Verification items for the finished model (mm, model axes). Face numbers are marked on the shaded views. Round coordinates to 2 decimals unless told otherwise and drop trailing zeros. Order: outer loops, then holes, each group sorted by start corner. A loop starts at its lowest first (then second) coordinate and runs counter-clockwise, first axis right, second up. Notation, with made-up numbers: (25.25, -25) -> (54.25, -25) arc R30 ccw to (54.25, -1) -> close; hole circle Ø3 at (81, 35). An arc over 180 degrees is marked (long way). Return JSON: item names as keys, results as strings. Group by question number.
1) Draft check along Y on the marked faces 1, 2, 3 and 4. Enter one of: pulls with the +Y half, pulls with the -Y half, needs draft (parallel to the pull), parting line crosses it, or undercut.
2) Section check A-A on y = 49.5. Enter the section's corners in (x, z) (3 decimals).
3) Scan lines: L1, parallel to Z at x = 2.25, y = 44 (3 decimals); L2, parallel to Z at x = 3.75, y = 17; L3, parallel to Y at x = 4.25, z = 9. Record each from-to range of solid material in increasing order.
4) Depth check by flat-ended pin: pin 1 (0.5 mm diameter, centred on x = 4, z = 3.5, fed in from +Y); pin 2 (4 mm diameter, centred on y = 18.5, z = 18, fed in from +X); pin 3 (1 mm diameter, centred on x = 6, z = 19.5, fed in from -Y); pin 4 (0.5 mm diameter, centred on x = 4, y = 17, fed in from -Z). Enter the tip coordinate at first touch or a pass-through.
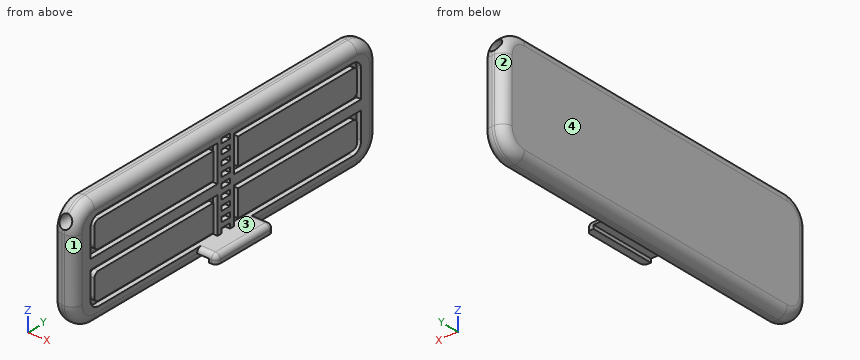
```python
from build123d import *

# Parameters (mm, degrees)
F1_DEPTH     = 4.5
F2_R         = 1.225
F3_DEPTH     = 74
F4_T1_DEPTH  = 64
F4_T3_DEPTH  = 13
F4_T6_ANGLE  = 90
F4_T8_ANGLE  = 90
F4_T10_ANGLE = 90
F4_T12_ANGLE = 90
F4_T14_ANGLE = 90
F4_T16_ANGLE = 90
F4_T18_ANGLE = 90
F4_T20_ANGLE = 90
F6_DEPTH     = 1
F7_W         = 2
F7_H         = 1
F8_DEPTH     = 1
F10_DEPTH    = 1
F11_W        = 14
F11_H        = 1
F12_DEPTH    = 4
F13_W        = 1.5
F13_H        = 14
F14_DEPTH    = 0.75
F15_R        = 0.99999


# Not quite as in the source:
# - a fillet or chamfer that OpenCascade refuses, or shapes differently, is made with other operations: its cross-section is extruded or revolved along the edge and cut away or added
# - a fillet or chamfer is up to 0.001 mm smaller than in the source, because OpenCascade refuses the exact size


with BuildPart() as f1:
    # F0 (on Right) → F1 (new body)
    with BuildSketch(Plane.YZ):
        with BuildLine():
            ThreePointArc((0, 5), (1.4644660941, 1.4644660941), (5, 0))
            Line((5, 0), (69, 0))
            ThreePointArc((69, 0), (72.5355339059, 1.4644660941), (74, 5))
            Line((74, 5), (74, 18))
            ThreePointArc((74, 18), (72.5355339059, 21.5355339059), (69, 23))
            Line((69, 23), (5, 23))
            ThreePointArc((5, 23), (1.4644660941, 21.5355339059), (0, 18))
            Line((0, 18), (0, 5))
        make_face()
    extrude(amount=F1_DEPTH)

    # F2 (on face) → F3 (cut, through all)
    with BuildSketch(Plane(origin=(0, 74, 0), x_dir=(-1, 0, 0), z_dir=(0, 1, 0))):
        with Locations((-2.25, 20)):
            Circle(F2_R)
    extrude(amount=-F3_DEPTH, mode=Mode.SUBTRACT)

    # F4: fillet of radius 2 on 16 edges, made by hand

    # F4_s2 → F4_t1 (cut)
    with BuildSketch(Plane.XZ.offset(-69)):
        with BuildLine():
            ThreePointArc((0, 21), (0.5857864376, 22.4142135624), (2, 23))
            Line((2, 23), (0, 23))
            Line((0, 23), (0, 21))
        make_face()
        with BuildLine():
            ThreePointArc((4.5, 21), (3.9142135624, 22.4142135624), (2.5, 23))
            Line((2.5, 23), (4.5, 23))
            Line((4.5, 23), (4.5, 21))
        make_face()
        with BuildLine():
            ThreePointArc((2, 0), (0.5857864376, 0.5857864376), (0, 2))
            Line((0, 2), (0, 0))
            Line((0, 0), (2, 0))
        make_face()
        with BuildLine():
            ThreePointArc((2.5, 0), (3.9142135624, 0.5857864376), (4.5, 2))
            Line((4.5, 2), (4.5, 0))
            Line((4.5, 0), (2.5, 0))
        make_face()
    extrude(amount=F4_T1_DEPTH, mode=Mode.SUBTRACT)

    # F4_s4 → F4_t3 (cut)
    with BuildSketch(Plane.XY.offset(5)):
        with BuildLine():
            ThreePointArc((2, 0), (0.5857864376, 0.5857864376), (0, 2))
            Line((0, 2), (0, 0))
            Line((0, 0), (2, 0))
        make_face()
        with BuildLine():
            ThreePointArc((2.5, 0), (3.9142135624, 0.5857864376), (4.5, 2))
            Line((4.5, 2), (4.5, 0))
            Line((4.5, 0), (2.5, 0))
        make_face()
        with BuildLine():
            ThreePointArc((0, 72), (0.5857864376, 73.4142135624), (2, 74))
            Line((2, 74), (0, 74))
            Line((0, 74), (0, 72))
        make_face()
        with BuildLine():
            ThreePointArc((4.5, 72), (3.9142135624, 73.4142135624), (2.5, 74))
            Line((2.5, 74), (4.5, 74))
            Line((4.5, 74), (4.5, 72))
        make_face()
    extrude(amount=F4_T3_DEPTH, mode=Mode.SUBTRACT)

    # F4_s5 → F4_t6 (revolve, cut)
    with BuildSketch(Plane.XY.offset(5)):
        with BuildLine():
            ThreePointArc((2, 0), (0.5857864376, 0.5857864376), (0, 2))
            Line((0, 2), (0, 0))
            Line((0, 0), (2, 0))
        make_face()
    revolve(axis=Axis((0, 5, 5), (1, 0, 0)), revolution_arc=F4_T6_ANGLE, mode=Mode.SUBTRACT)

    # F4_s7 → F4_t8 (revolve, cut)
    with BuildSketch(Plane.XY.offset(5)):
        with BuildLine():
            ThreePointArc((2.5, 0), (3.9142135624, 0.5857864376), (4.5, 2))
            Line((4.5, 2), (4.5, 0))
            Line((4.5, 0), (2.5, 0))
        make_face()
    revolve(axis=Axis((4.5, 5, 5), (1, 0, 0)), revolution_arc=F4_T8_ANGLE, mode=Mode.SUBTRACT)

    # F4_s9 → F4_t10 (revolve, cut)
    with BuildSketch(Plane.XZ.offset(-69)):
        with BuildLine():
            ThreePointArc((0, 2), (0.5857864376, 0.5857864376), (2, 0))
            Line((2, 0), (0, 0))
            Line((0, 0), (0, 2))
        make_face()
    revolve(axis=Axis((0, 69, 5), (1, 0, 0)), revolution_arc=F4_T10_ANGLE, mode=Mode.SUBTRACT)

    # F4_s11 → F4_t12 (revolve, cut)
    with BuildSketch(Plane.XY.offset(18)):
        with BuildLine():
            ThreePointArc((0, 72), (0.5857864376, 73.4142135624), (2, 74))
            Line((2, 74), (0, 74))
            Line((0, 74), (0, 72))
        make_face()
    revolve(axis=Axis((0, 69, 18), (1, 0, 0)), revolution_arc=F4_T12_ANGLE, mode=Mode.SUBTRACT)

    # F4_s13 → F4_t14 (revolve, cut)
    with BuildSketch(Plane.XZ.offset(-5)):
        with BuildLine():
            ThreePointArc((0, 21), (0.5857864376, 22.4142135624), (2, 23))
            Line((2, 23), (0, 23))
            Line((0, 23), (0, 21))
        make_face()
    revolve(axis=Axis((0, 5, 18), (1, 0, 0)), revolution_arc=F4_T14_ANGLE, mode=Mode.SUBTRACT)

    # F4_s15 → F4_t16 (revolve, cut)
    with BuildSketch(Plane.XZ.offset(-69)):
        with BuildLine():
            ThreePointArc((4.5, 2), (3.9142135624, 0.5857864376), (2.5, 0))
            Line((2.5, 0), (4.5, 0))
            Line((4.5, 0), (4.5, 2))
        make_face()
    revolve(axis=Axis((4.5, 69, 5), (1, 0, 0)), revolution_arc=F4_T16_ANGLE, mode=Mode.SUBTRACT)

    # F4_s17 → F4_t18 (revolve, cut)
    with BuildSketch(Plane.XY.offset(18)):
        with BuildLine():
            ThreePointArc((4.5, 72), (3.9142135624, 73.4142135624), (2.5, 74))
            Line((2.5, 74), (4.5, 74))
            Line((4.5, 74), (4.5, 72))
        make_face()
    revolve(axis=Axis((4.5, 69, 18), (1, 0, 0)), revolution_arc=F4_T18_ANGLE, mode=Mode.SUBTRACT)

    # F4_s19 → F4_t20 (revolve, cut)
    with BuildSketch(Plane.XZ.offset(-5)):
        with BuildLine():
            ThreePointArc((4.5, 21), (3.9142135624, 22.4142135624), (2.5, 23))
            Line((2.5, 23), (4.5, 23))
            Line((4.5, 23), (4.5, 21))
        make_face()
    revolve(axis=Axis((4.5, 5, 18), (1, 0, 0)), revolution_arc=F4_T20_ANGLE, mode=Mode.SUBTRACT)

    # F5 (on face) → F6 (cut)
    with BuildSketch(Plane.YZ.offset(4.5)):
        with BuildLine():
            Line((35, 20), (6, 20))
            ThreePointArc((6, 20), (4.5857864376, 19.4142135624), (4, 18))
            Line((4, 18), (4, 12.5))
            Line((4, 12.5), (35, 12.5))
            Line((35, 12.5), (35, 20))
        make_face()
        with BuildLine():
            ThreePointArc((4, 5), (4.5857864376, 3.5857864376), (6, 3))
            Line((6, 3), (35, 3))
            Line((35, 3), (35, 10.5))
            Line((35, 10.5), (4, 10.5))
            Line((4, 10.5), (4, 5))
        make_face()
        with BuildLine():
            Line((68, 20), (39, 20))
            Line((39, 20), (39, 12.5))
            Line((39, 12.5), (70, 12.5))
            Line((70, 12.5), (70, 18))
            ThreePointArc((70, 18), (69.4142135624, 19.4142135624), (68, 20))
        make_face()
        with BuildLine():
            Line((39, 10.5), (39, 3))
            Line((39, 3), (68, 3))
            ThreePointArc((68, 3), (69.4142135624, 3.5857864376), (70, 5))
            Line((70, 5), (70, 10.5))
            Line((70, 10.5), (39, 10.5))
        make_face()
    extrude(amount=-F6_DEPTH, mode=Mode.SUBTRACT)

    # F7 (on face) → F8 (cut)
    with BuildSketch(Plane.YZ.offset(4.5)):
        with Locations((37, 3.5)):
            Rectangle(F7_W, F7_H)
        with Locations((37, 5.56)):
            Rectangle(F7_W, F7_H)
        with Locations((37, 7.62)):
            Rectangle(F7_W, F7_H)
        with Locations((37, 9.68)):
            Rectangle(F7_W, F7_H)
        with Locations((37, 11.74)):
            Rectangle(F7_W, F7_H)
        with Locations((37, 13.8)):
            Rectangle(F7_W, F7_H)
        with Locations((37, 15.86)):
            Rectangle(F7_W, F7_H)
        with Locations((37, 17.92)):
            Rectangle(F7_W, F7_H)
        with Locations((37, 19.98)):
            Rectangle(F7_W, F7_H)
    extrude(amount=-F8_DEPTH, mode=Mode.SUBTRACT)

    # F9 (on face) → F10 (join)
    with BuildSketch(Plane.YZ.offset(3.5)):
        with BuildLine():
            ThreePointArc((5, 5), (5.2928932188, 4.2928932188), (6, 4))
            Line((6, 4), (34, 4))
            Line((34, 4), (34, 9.5))
            Line((34, 9.5), (6, 9.5))
            ThreePointArc((6, 9.5), (5.2928932188, 9.2071067812), (5, 8.5))
            Line((5, 8.5), (5, 5))
        make_face()
        with BuildLine():
            Line((34, 19), (6, 19))
            ThreePointArc((6, 19), (5.2928932188, 18.7071067812), (5, 18))
            Line((5, 18), (5, 14.5))
            ThreePointArc((5, 14.5), (5.2928932188, 13.7928932188), (6, 13.5))
            Line((6, 13.5), (34, 13.5))
            Line((34, 13.5), (34, 19))
        make_face()
        with BuildLine():
            ThreePointArc((69, 8.5), (68.7071067812, 9.2071067812), (68, 9.5))
            Line((68, 9.5), (40, 9.5))
            Line((40, 9.5), (40, 4))
            Line((40, 4), (68, 4))
            ThreePointArc((68, 4), (68.7071067812, 4.2928932188), (69, 5))
            Line((69, 5), (69, 8.5))
        make_face()
        with BuildLine():
            ThreePointArc((68, 13.5), (68.7071067812, 13.7928932188), (69, 14.5))
            Line((69, 14.5), (69, 18))
            ThreePointArc((69, 18), (68.7071067812, 18.7071067812), (68, 19))
            Line((68, 19), (40, 19))
            Line((40, 19), (40, 13.5))
            Line((40, 13.5), (68, 13.5))
        make_face()
    extrude(amount=F10_DEPTH)

    # F11 (on face) → F12 (join)
    with BuildSketch(Plane.YZ.offset(4.5)):
        with Locations((37, 2.5)):
            Rectangle(F11_W, F11_H)
    extrude(amount=F12_DEPTH)

    # F13 (on face) → F14 (join)
    with BuildSketch(Plane(origin=(0, 0, 2), x_dir=(1, 0, 0), z_dir=(0, 0, -1))):
        with Locations((7.75, -37)):
            Rectangle(F13_W, F13_H)
    extrude(amount=F14_DEPTH)

    # F15 (radius 1 in the source; OpenCascade refuses exactly that, so slightly less here)
    f15_edges = [f1.edges().sort_by_distance(p)[0] for p in [
        (8.5, 37, 3),
        (6.5, 30, 3),
        (6.5, 44, 3),
        (8.5, 44, 2.125),
        (8.5, 30, 2.125),
    ]]
    fillet(f15_edges, radius=F15_R)


solid = f1.part
```
Check result:
{
 "1": {"face 1": "pulls with the -Y half", "face 2": "pulls with the +Y half", "face 3": "undercut", "face 4": "needs draft"},
 "2": {"outline": "(0, 2) arc R2 ccw to (2, 0) -> (2.5, 0) arc R2 ccw to (4.5, 2) -> (4.5, 3) -> (3.5, 3) -> (3.5, 4) -> (4.5, 4) -> (4.5, 9.5) -> (3.5, 9.5) -> (3.5, 10.5) -> (4.5, 10.5) -> (4.5, 12.5) -> (3.5, 12.5) -> (3.5, 13.5) -> (4.5, 13.5) -> (4.5, 19) -> (3.5, 19) -> (3.5, 20) -> (4.5, 20) -> (4.5, 21) arc R2 ccw to (2.5, 23) -> (2, 23) arc R2 ccw to (0, 21) -> close; hole circle Ø2.45 at (2.25, 20)"},
 "3": {"L1": "0 to 18.775, 21.225 to 23", "L2": "0.44 to 3, 4 to 9.5, 10.5 to 12.5, 13.5 to 19, 20 to 22.56", "L3": "1.03 to 4, 5.13 to 34, 35 to 39, 40 to 68.87, 70 to 72.97"},
 "4": {"pin 1": "y = 73.32", "pin 2": "x = 4.5", "pin 3": "through", "pin 4": "z = 0.44"}
}
